from build123d import *

# Parameters (mm, degrees)
F0_W     = 17.9
F0_H     = 12.3
F1_DEPTH = 6.9
F2_R     = 4.1
F3_DEPTH = 1.1
F7_R     = 3.675
F4_R     = 4.3


with BuildPart() as f1:
    # F0 (on Top) → F1 (new body)
    with BuildSketch(Plane.XY):
        Rectangle(F0_W, F0_H)
    extrude(amount=F1_DEPTH)

    # F2 (on face) → F3 (join)
    with BuildSketch(Plane.XY.offset(6.9)):
        Circle(F2_R)
    extrude(amount=F3_DEPTH)

    # F7 (on plane+point) → F8 section 0
    with BuildSketch(Plane.XY.offset(12.4)):
        Circle(F7_R)
    # F4 (on face) → F8 section 1
    with BuildSketch(Plane.XY.offset(8)):
        Circle(F4_R)
    loft()


solid = f1.part
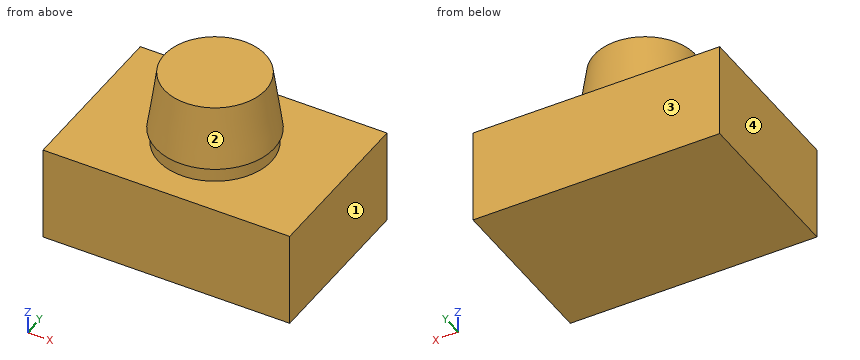
Here's how the part is built. I have some questions about the finished solid (model axes, mm). Face numbers are marked on the shaded views. Round coordinates to 2 decimals unless told otherwise and drop trailing zeros. Write each loop counter-clockwise with the first axis right and the second up, starting at its lowest first coordinate (ties: lowest second). Pieces come first, ordered by that corner, then holes.
1. Suppose I cut it at A-A (x = 0). List the corners of the cut face in (y, z) for me (3 decimals), and give its area (3 significant figures).
2. Suppose I cut it at C-C (x = -5.25). List the corners of the cut face in (y, z) for me, and give its area (3 significant figures).
3. I need wall thicknesses on L1, parallel to Z at x = 7.5, y = 5.5; L2, parallel to Y at x = 2, z = 10.25; L3, parallel to X at y = 1.5, z = 10.25. Which ranges of each line are inside material? Lowest first, please.
4. Will this pin go through, and if not, where does the flat tip stop? pin 1 Ø4 at (x, y) = (4, 1.5) entering from -Z.
5. Suppose I cut it at D-D (z = 9.75). List the corners of the cut face in (x, y) for me, and give its area (3 significant figures).
6. Suppose I cut it at B-B (z = 8.5). List the corners of the cut face in (x, y) for me.
7. If we mould it in two halves opening along X, with no side actions, what happens to the marked faces 1, 2, 3 and 4? For each: released by +X, released by -X, zero draft, split by the parting line, or undercut.
Answer sheet:
1. outline: (-6.15, 0) - (6.15, 0) - (6.15, 6.9) - (4.1, 6.9) - (4.1, 8) - (4.3, 8) - (3.675, 12.4) - (-3.675, 12.4) - (-4.3, 8) - (-4.1, 8) - (-4.1, 6.9) - (-6.15, 6.9) - close
1. area: 129 mm2
2. outline: (-6.15, 0) - (6.15, 0) - (6.15, 6.9) - (-6.15, 6.9) - close
2. area: 84.9 mm2
3. L1: z = 0 to 6.9
3. L2: y = -3.44 to 3.44
3. L3: x = -3.69 to 3.69
4. pin 1: stops at z = 0
5. outline: circle Ø8.1 at (0, 0)
5. area: 51.6 mm2
6. outline: circle Ø8.46 at (0, 0)
7. face 1: released by +X
7. face 2: split by the parting line
7. face 3: zero draft
7. face 4: released by -X
